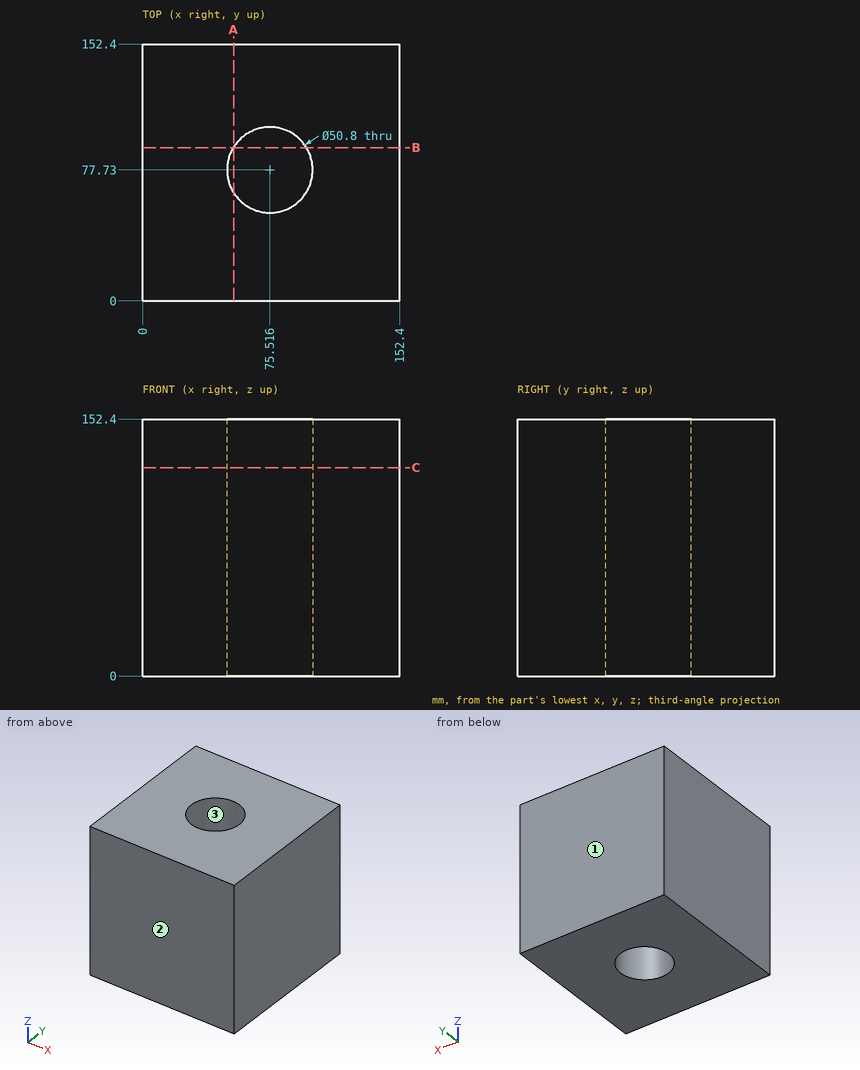
Study the drawing (mm; zero at the part's minimum x, y, z) and answer. Give positions to 0.01 mm unless a question says otherwise; leave off trailing zeros. Order: outer loops, then holes, each group sorted by start corner. A loop starts at its lowest first (then second) coordinate and runs counter-clockwise, first axis right, second up. Notation, with made-up numbers: (48.5, 71) - (81.5, 71) arc R18 cw to (81.5, 93) - close; hole circle Ø11 at (1.25, 3.25). An arc over 180 degrees is marked (long way). Use one line per item in the form item = value. Start each with the question number.
(1) The mould has two halves that part along Y. Classify the marked faces 1, 2 and 3: released by +Y, released by -Y, zero draft, split by the parting line, or undercut.
(2) A cutting plane is placed at A-A, the plane x = 54. Write down the section's boundary in (y, z), then the cut area to 3 significant figures.
(3) A cutting plane is placed at B-B, the plane y = 91. Write down the section's boundary in (x, z) (1 decimal), then the cut area to 3 significant figures.
(4) Consider line 1 (X direction, y = 58, z = 95) (1 decimal); line 2 (X direction, y = 69.5, z = 90.5) (1 decimal); line 3 (Y direction, x = 96, z = 109). Determine where each line is inside the solid, lowest interval first. Write a range as from..to.
(5) A cutting plane is placed at C-C, the plane z = 123.5. Write down the section's boundary in (x, y).
Ans:
q1.face_1 = released by +Y
q1.face_2 = released by -Y
q1.face_3 = undercut
q2.outline = (0, 0) - (64.23, 0) - (64.23, 152.4) - (0, 152.4) - close; (91.23, 0) - (152.4, 0) - (152.4, 152.4) - (91.23, 152.4) - close
q2.area = 19,100 mm^2
q3.outline = (0, 0) - (53.9, 0) - (53.9, 152.4) - (0, 152.4) - close; (97.2, 0) - (152.4, 0) - (152.4, 152.4) - (97.2, 152.4) - close
q3.area = 16,600 mm^2
q4.line_1 = 0..59.5, 91.5..152.4
q4.line_2 = 0..51.5, 99.5..152.4
q4.line_3 = 0..62.71, 92.75..152.4
q5.outline = (0, 0) - (152.4, 0) - (152.4, 152.4) - (0, 152.4) - close; hole circle Ø50.8 at (75.52, 77.73)
